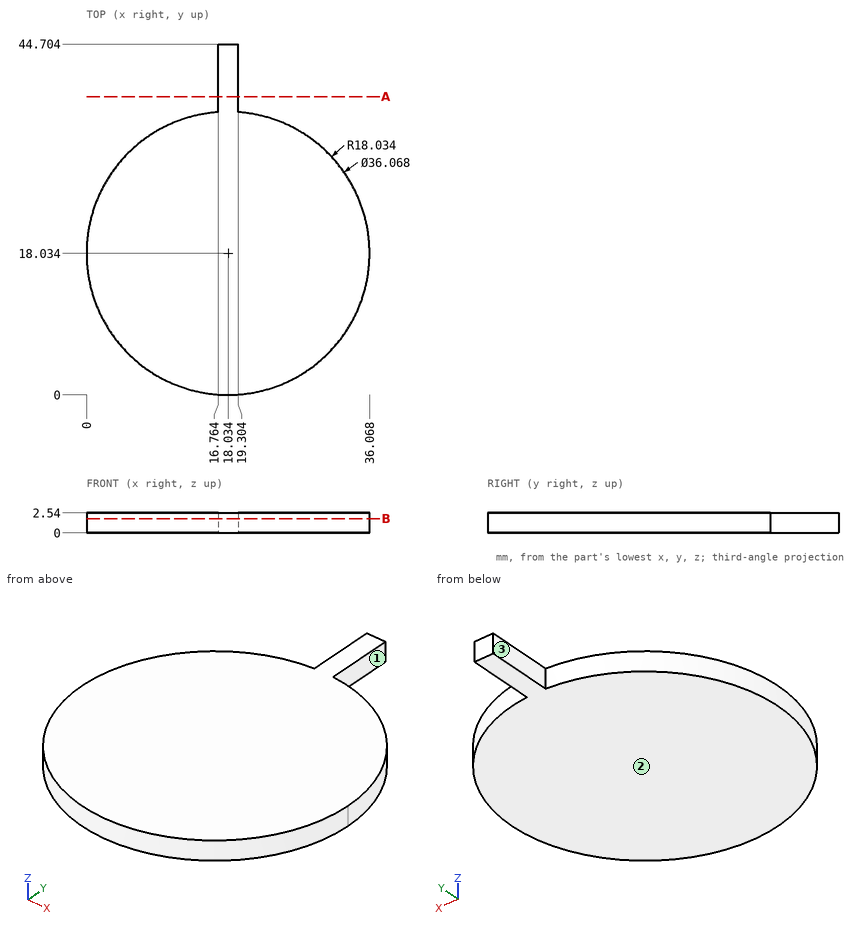
The drawing under review shows one solid part. Ordinate dimensions are in mm from its lowest x, y, z. A direction names the side the tool comes from. Give positions to 0.01 mm unless a question says otherwise; leave off trailing zeros. Write each loop counter-clockwise with the first axis right and the second up, starting at its lowest first coordinate (ties: lowest second). Pieces come first, ordered by that corner, then holes.
1. Add section A-A, the plane y = 38. Write out the cut boundary in (x, z).
2. For P1, Ø1.5, axis at x = 11, z = 0.5, coming from the -Y side; P2, Ø1, axis at y = 25, z = 1.5, coming from the -X side; P3, Ø1.5, axis at y = 12, z = 1, coming from the +X side, all flat-tipped, find the tip position at first contact; note any pin that passes through.
3. Wall thickness on L1, parallel to X at y = 41, z = 1.2; L2, parallel to Y at x = 18.5, z = 1.25; L3, parallel to X at y = 32.5, z = 1.4: over which ranges is each line inside the solid? List them lowest first.
4. Tool access review of the marked faces 1, 2 and 3: name each direction out of +Z, -Z, +X, -X, +Y, -Y from which nothing blocks a thin tool from reaching the whole face with its end or side.
5. Add section B-B, the plane z = 1.8. Write out the cut boundary in (x, y), plus the area to 3 significant figures.
Worked answers:
1. outline: (16.76, 0) - (19.3, 0) - (19.3, 2.54) - (16.76, 2.54) - close
2. P1: stops at y = 1.13
2. P2: stops at x = 1.2
2. P3: stops at x = 35.28
3. L1: x = 16.76 to 19.3
3. L2: y = 0.01 to 44.7
3. L3: x = 7.27 to 28.8
4. face 1: +Z, -Z, +X, +Y
4. face 2: -Z, +X, -X, +Y, -Y
4. face 3: +Z, -Z, -X, +Y
5. outline: (16.76, 36.02) arc R18.03 ccw (long way) to (19.3, 36.02) - (19.3, 44.7) - (16.76, 44.7) - close
5. area: 1,040 mm2
